```python
from build123d import *

# Parameters (mm, degrees)
F1_DEPTH  = 50.8
F2_R      = 16.9023108292
F2_R_2    = 15.9336293425
F3_DEPTH  = 25.4
F4_W      = 6.4683202654
F4_H      = 8.9478455484
F5_DEPTH  = 20.1422
F7_DEPTH  = 20.1422
F9_DEPTH  = 5.08
F11_DEPTH = 5.08
F13_DEPTH = 5.08


with BuildPart() as f1:
    # F0 (on Front) → F1 (new body)
    with BuildSketch(Plane.XZ):
        with BuildLine():
            Line((10.3610064834, 27.9171578586), (-10.9366187826, 27.9171578586))
            Line((-10.9366187826, 27.9171578586), (-10.9366187826, 48.0635650456))
            add(Edge.make_bspline(
                [(-69.6489959955, 0), (-71.3521609697, 9.1404972773), (-75.7031147589, 32.4910721582), (-35.4393063841, 42.172124994), (-10.9366187826, 48.0635650456)],
                knots=[0, 0, 0, 0, 0.3914463487, 1, 1, 1, 1], degree=3))
            add(Edge.make_bspline(
                [(-69.6489959955, 0), (-65.6808981625, -9.7567834982), (-56.8491666777, -31.4722995051), (-1.4859571576, -29.3762186894), (0, -30.5074099451)],
                knots=[0, 0, 0, 0, 0.4310565027, 0.9593955207, 0.9593955207, 0.9593955207, 0.9593955207], degree=3))
            add(Edge.make_bspline(
                [(0, -30.5074099451), (20.8319398692, -31.1069128662), (56.9844176124, -32.1473112232), (65.2730555247, -9.5683941039), (68.7855780125, 0)],
                knots=[0, 0, 0, 0, 0.576224402, 1, 1, 1, 1], degree=3))
            add(Edge.make_bspline(
                [(10.3610064834, 48.0635650456), (30.289884659, 42.7388235814), (64.8673270211, 33.5001730438), (67.6195937052, 9.968906062), (68.7855780125, 0)],
                knots=[0, 0, 0, 0, 0.5763548954, 1, 1, 1, 1], degree=3))
            Line((10.3610064834, 48.0635650456), (10.3610064834, 27.9171578586))
        make_face()
    extrude(amount=F1_DEPTH)

    # F2 (on face) → F3 (cut)
    with BuildSketch(Plane.XZ.offset(50.8)):
        with Locations((-39.7171936929, 7.4829496443)):
            Circle(F2_R)
        with Locations((36.5513339639, 7.4829496443)):
            Circle(F2_R_2)
    extrude(amount=-F3_DEPTH, mode=Mode.SUBTRACT)

    # F4 (on Top) → F5 (cut)
    with BuildSketch(Plane.XY):
        with Locations((-14.1248302534, -29.9614351243)):
            Rectangle(F4_W, F4_H)
        Polygon((17.0188006014, -25.4875123501), (10.3522520512, -25.4875123501), (10.4804551229, -34.4353578985), (17.0188006014, -34.4353578985), align=None)
    extrude(amount=-F5_DEPTH, mode=Mode.SUBTRACT)

    # F6 (on Top) → F7 (cut)
    with BuildSketch(Plane.XY):
        Polygon((-10.9366187826, -33.3854667842), (-11.2244244665, -20.4342082143), (-22.1610441804, -20.4342082143), (-22.1610441804, -33.3854667842), align=None)
        Polygon((21.8732375652, -20.4342082143), (10.0732007995, -20.4342082143), (10.3610064834, -33.3854667842), (21.8732375652, -33.3854667842), align=None)
    extrude(amount=-F7_DEPTH, mode=Mode.SUBTRACT)

    # F8 (on face) → F9 (cut)
    with BuildSketch(Plane.YZ.offset(-10.9366187826)):
        Polygon((-32.5317271054, 27.9171578586), (-25.4, 48.0635650456), (-32.5317271054, 48.0635650456), (-42.7853837609, 27.9171578586), align=None)
    extrude(amount=-F9_DEPTH, mode=Mode.SUBTRACT)

    # F10 (on Front) → F11 (cut)
    with BuildSketch(Plane.XZ):
        Polygon((29.1642211378, 44.9136085808), (20.9452454001, 46.1828112602), (29.1642211378, 24.8657949269), (35.5472825468, 23.4038140625), align=None)
    extrude(amount=-F11_DEPTH, mode=Mode.SUBTRACT)

    # F12 (on face) → F13 (cut)
    with BuildSketch(Plane(origin=(10.3610064834, 0, 0), x_dir=(0, -1, 0), z_dir=(-1, 0, 0))):
        Polygon((33.6429066956, 48.0635650456), (27.8411041945, 48.0635650456), (41.0764664412, 27.9171578586), (46.6969534755, 27.9171578586), align=None)
    extrude(amount=-F13_DEPTH, mode=Mode.SUBTRACT)


solid = f1.part
```
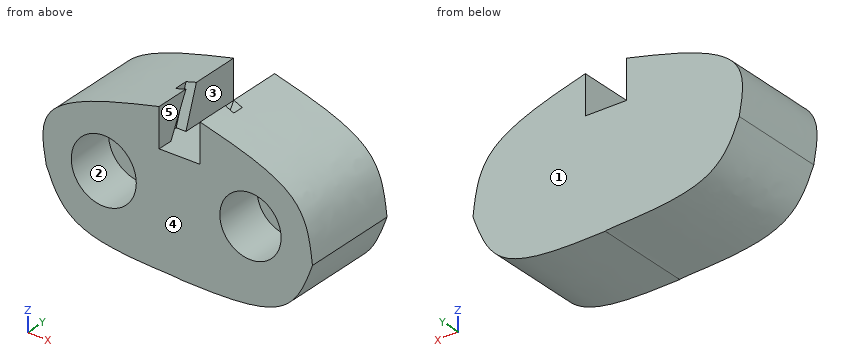
Can you work these out from the model? Positions are in its coordinate system, mm. Face numbers are marked on the shaded views. A direction names the side the tool comes from. Coordinates: 2 decimals unless noted, no trailing zeros.
1) Which directions (+Z, -Z, +X, -X, +Y, -Y) give clear straight access to the entire face, cutting with the end or side of a thin tool? Please do the marked faces 1, 2 and 3.
2) For pin 1 (22 mm diameter, centred on y = -24, z = 42.5, fed in from +X); pin 2 (14.5 mm diameter, centred on y = -33, z = 40, fed in from -X); pin 3 (7 mm diameter, centred on y = -31, z = -13.5, fed in from -X), each with a flat end and sliding along its axis, tell me the tip position at first contact or that it passes through.
3) Thinking about a two-plate mould opening in X: for the marked faces 4 and 5, which applies, pulls with the +X half, pulls with the -X half, needs draft (parallel to the pull), parting line crosses it, or undercut?
4) Imagine slicing it at A-A on y = -44.5. State how many separate pieces and enclosed holes the cut face has, plus the area to 3 significant figures.
5) I need wall thicknesses on probe 1 along Y at (x, z) = (-15, -11); probe 2 along X at (y, z) = (-35, 19); probe 3 along X at (y, z) = (-34, 11.5). Which ranges of each line are inside material? Lowest first, please.
Completed:
1. face 1: +Z, -Z, +X, -X, +Y
1. face 2: -Y
1. face 3: +Z, +Y, -Y
2. pin 1: stops at x = 54.78
2. pin 2: stops at x = -58.96
2. pin 3: stops at x = -65.1
3. face 4: needs draft
3. face 5: undercut
4. separate pieces: 1
4. enclosed holes: 2
4. area: 6,880 mm2
5. probe 1: y = -50.8 to -34.44, -20.43 to 0
5. probe 2: x = -70.77 to -52.09, -27.35 to 25.54, 47.56 to 64.84
5. probe 3: x = -71.3 to -56.14, -23.3 to 21.13, 51.97 to 67.08
